from build123d import *

# Parameters (mm, degrees)
SKETCH_1_R          = 7
SKETCH_1_R_2        = 1.5
EXTRUDE_1_DEPTH     = 3
CUT_EXTRUDE_1_DEPTH = 2


with BuildPart() as part:
    # Эскиз1 → Бобышка-Вытянуть1 (new body)
    with BuildSketch(Plane(origin=(0, 0, 0), x_dir=(1, 0, 0), z_dir=(0, 1, 0))):
        with Locations(Location((0, 0, 0), (0, 0, 270))):
            Circle(SKETCH_1_R)
        with Locations(Location((0, 0, 0), (0, 0, 270))):
            Circle(SKETCH_1_R_2, mode=Mode.SUBTRACT)
    extrude(amount=EXTRUDE_1_DEPTH)

    # Эскиз2 → Вырез-Вытянуть1 (cut)
    with BuildSketch(Plane(origin=(0, 3, 0), x_dir=(1, 0, 0), z_dir=(0, 1, 0))):
        Polygon((1.58771324, 2.75), (-1.58771324, 2.75), (-3.175426481, 0), (-1.58771324, -2.75), (1.58771324, -2.75), (3.175426481, 0), align=None)
    extrude(amount=-CUT_EXTRUDE_1_DEPTH, mode=Mode.SUBTRACT)


solid = part.part
Here's how the part is built. I have some questions about the finished solid (model axes, mm). A direction names the side the tool comes from. Round coordinates to 2 decimals unless told otherwise and drop trailing zeros. Order: outer loops, then holes, each group sorted by start corner. A loop starts at its lowest first (then second) coordinate and runs counter-clockwise, first axis right, second up. Notation, with made-up numbers: M 56,49 L 86,49 A16 cw 86,60 Z; hole C 67,37.5 d2. An arc over 180 degrees is marked long. One line per question, with ' | ' between items.
1) I need wall thicknesses on line 1 (X direction, y = 0.35, z = 0); line 2 (Y direction, x = -2.75, z = 0.25); line 3 (Z direction, x = -0.25, y = 1.3). Which ranges of each line are inside material? Lowest first, please.
Checked values:
line 1: x = -7 to -1.5, 1.5 to 7 | line 2: y = 0 to 1 | line 3: z = -7 to -2.75, 2.75 to 7
2) Imagine slicing it at B-B, the plane y = 1.7. Write out the boundary of the cut face in (x, z).
Checked values:
outline: C 0,0 d14; hole M -3.18,0 L -1.59,-2.75 L 1.59,-2.75 L 3.18,0 L 1.59,2.75 L -1.59,2.75 Z
3) On a 3-axis mill with a long thin cutter (end or side, diameter ignored), from which of +Z, -Z, +X, -X, +Y, -Y can I reach the whole of each face in a straight line? I mean faces 5 (the flat face through (-2.37, 2.014, -1.394)), 6 (the cylindrical face through (0.45, 0.49, 1.43)). Say none if no direction works.
Checked values:
face 5: +Y | face 6: +Y, -Y
4) Imagine slicing it at A-A, the plane x = 0. Write out the boundary of the cut face in (y, z), plus the area to 3 significant figures.
Checked values:
outline: M 0,-7 L 3,-7 L 3,-2.75 L 1,-2.75 L 1,-1.5 L 0,-1.5 Z; M 0,1.5 L 1,1.5 L 1,2.75 L 3,2.75 L 3,7 L 0,7 Z | area: 28.0 mm²
5) Imagine slicing it at D-D, the plane y = 0.7. Write out the boundary of the cut face in (x, z).
Checked values:
outline: C 0,0 d14; hole C 0,0 d3
6) Imagine slicing it at C-C, the plane z = 2. Write out the boundary of the cut face in (x, y).
Checked values:
outline: M -6.71,0 L 6.71,0 L 6.71,3 L 2.02,3 L 2.02,1 L -2.02,1 L -2.02,3 L -6.71,3 Z
7) I'm going to push flat-ended pins straight in: pin 1 Ø1.5 at (y, z) = (1, -4.5) entering from +X; pin 2 Ø1.6 at (x, z) = (1.5, 1) entering from +Y; pin 3 Ø1 at (x, z) = (1, 3) entering from -Y; pin 4 Ø1.5 at (y, z) = (2.5, 1.5) entering from +X. Where does each tip first touch, or does it pass through?
Checked values:
pin 1: stops at x = 5.91 | pin 2: stops at y = 1 | pin 3: stops at y = 0 | pin 4: stops at x = 6.96
8) We'd pull the mould along X, two halves only. Please class faces 1 (the flat face through (2.39, 2.01, -1.36)), 2 (the flat face through (2.37, 2.014, 1.394)), 3 (the flat face through (2, 0, 0)), 4 (the cylindrical face through (-6.834, 1.479, -1.517)): released by +X, released by -X, zero draft, split by the parting line, or undercut.
Checked values:
face 1: undercut | face 2: undercut | face 3: zero draft | face 4: split by the parting line
